Verification items for the finished model (mm, model axes). A direction names the side the tool comes from. Round coordinates to 2 decimals unless told otherwise and drop trailing zeros. Loops run counter-clockwise (first coordinate to the right, second up) from the corner with the lowest first, then second, coordinate; pieces in that order, holes last. Notation, with made-up numbers: (43.25, 24) - (75.25, 24) arc R17 ccw to (75.25, 55) - close; hole circle Ø11 at (-38, -12). An arc over 180 degrees is marked (long way). Use CSV: the item, a comma, the result in double quotes.
```python
from build123d import *

# Parameters (mm, degrees)
SKETCH1_R             = 80
BOSS_EXTRUDE1_DEPTH   = 13
SKETCH2_R             = 27.5
CUT_EXTRUDE1_DEPTH    = 114.881517377
SKETCH3_R             = 1.77324001
CUT_EXTRUDE2_DEPTH    = 12.744098
CIRPATTERN1_START     = 0.255902499
CIRPATTERN1_OUTLINE_R = 1.77324001
CIRPATTERN1_DEPTH     = 12.744097501


# Read off the part's stored shape, not the designer's step: CirPattern1
with BuildPart() as part:
    # Sketch1 → Boss-Extrude1 (new body)
    with BuildSketch(Plane(origin=(0, 0, 0), x_dir=(1, 0, 0), z_dir=(0, 1, 0))):
        with Locations(Location((0, 0, 0), (0, 0, 90))):
            Circle(SKETCH1_R)
    extrude(amount=BOSS_EXTRUDE1_DEPTH)

    # Sketch2 → Cut-Extrude1 (cut, through all)
    with BuildSketch(Plane(origin=(0, 0, 0), x_dir=(1, 0, 0), z_dir=(0, 1, 0))):
        with Locations(Location((0, 0, 0), (0, 0, 90))):
            Circle(SKETCH2_R)
    extrude(amount=CUT_EXTRUDE1_DEPTH, mode=Mode.SUBTRACT)

    # Sketch3 → Cut-Extrude2 (cut)
    with BuildSketch(Plane(origin=(0, 13, 0), x_dir=(1, 0, 0), z_dir=(0, 1, 0))):
        with Locations(Location((-29.492361813, 0, 0), (0, 0, 270))):
            Circle(SKETCH3_R)
    extrude(amount=-CUT_EXTRUDE2_DEPTH, mode=Mode.SUBTRACT)

    # CirPattern1 outline → CirPattern1 (cut)
    with BuildSketch(Plane(origin=(0, 0, 0), x_dir=(1, 0, 0), z_dir=(0, 1, 0)).offset(CIRPATTERN1_START)):
        with Locations((-20.854249031, -20.854249031)):
            Circle(CIRPATTERN1_OUTLINE_R)
        with Locations((-20.854249031, 20.854249031)):
            Circle(CIRPATTERN1_OUTLINE_R)
        with Locations((0, 29.492361813)):
            Circle(CIRPATTERN1_OUTLINE_R)
        with Locations((20.854249031, 20.854249031)):
            Circle(CIRPATTERN1_OUTLINE_R)
        with Locations((29.492361813, 0)):
            Circle(CIRPATTERN1_OUTLINE_R)
        with Locations((20.854249031, -20.854249031)):
            Circle(CIRPATTERN1_OUTLINE_R)
        with Locations((0, -29.492361813)):
            Circle(CIRPATTERN1_OUTLINE_R)
    extrude(amount=CIRPATTERN1_DEPTH, mode=Mode.SUBTRACT)


solid = part.part
```
1) Cross-section at C-C, the plane y = 4.25. Count the separate pieces of the cut face and the enclosed holes in it, then the cut area to 3 significant figures.
Returned:
separate pieces,"1"
enclosed holes,"9"
area,"17,700 mm²"
2) Cross-section at A-A, the plane z = 10. Record the cut outline in (x, y).
Returned:
outline,"(-79.37, 0) - (-25.62, 0) - (-25.62, 13) - (-79.37, 13) - close; (25.62, 0) - (79.37, 0) - (79.37, 13) - (25.62, 13) - close"
3) Cross-section at B-B, the plane x = 8. Record the cut outline in (y, z), then the cut area to 3 significant figures.
Returned:
outline,"(0, -79.6) - (13, -79.6) - (13, -26.31) - (0, -26.31) - close; (0, 26.31) - (13, 26.31) - (13, 79.6) - (0, 79.6) - close"
area,"1,390 mm²"
4) Gauge pin test, flat ends, axial feed: pin 1 Ø1 at (x, y) = (28, 2) entering from +Z; pin 2 Ø1.5 at (y, z) = (11, -59.5) entering from +X; pin 3 Ø1.1 at (x, z) = (1, -30) entering from +Y. Record the tip position at first contact, or that the pin passes through.
Returned:
pin 1,"stops at z = 75.12"
pin 2,"stops at x = 54.3"
pin 3,"stops at y = 0.26"
5) Cross-section at D-D, the plane x = -62. Record the cut outline in (y, z).
Returned:
outline,"(0, -50.56) - (13, -50.56) - (13, 50.56) - (0, 50.56) - close"
6) Access from +Z, -Z, +X, -X, +Y, -Y to the whole of each face (thin tool, end or side, straight path). Record for faces 1 (the face through (24.397, 6.409, -12.69)), 2 (the face through (21, 0.256, -21)).
Returned:
face 1,"+Y, -Y"
face 2,"+Y"
7) Mould release check, pull along X, two halves, no side actions. Record for faces 3 (the face through (29, 0.256, 0)), 4 (the face through (0.818, 6.539, 31.066)), 5 (the face through (78.1, 6.41, 17.34)), 6 (the face through (-1, 13, -34)): +X half, -X half, draft (parallel to the pull), parting line (faces both ways), or undercut.
Returned:
face 3,"undercut"
face 4,"undercut"
face 5,"parting line"
face 6,"draft"
8) Thickness scan on probe 1 along X at (y, z) = (6.25, 0); probe 2 along Z at (x, y) = (-13.5, 11); probe 3 along Z at (x, y) = (-30, 11.5). Record the ranges inside material, lowest first. Write a range as [from, to].
Returned:
probe 1,"x = [-80, -31.27], [-27.72, -27.5], [27.5, 27.72], [31.27, 80]"
probe 2,"z = [-78.85, -23.96], [23.96, 78.85]"
probe 3,"z = [-74.16, -1.7], [1.7, 74.16]"
